Verification items for this drawing (mm, ordinates from the low corner). A direction names the side the tool comes from. Give positions to 0.01 mm unless a question says otherwise; leave off trailing zeros. Loops run counter-clockwise (first coordinate to the right, second up) from the corner with the lowest first, then second, coordinate; pieces in that order, holes last. Notation, with made-up numbers: (-10, 20.5) - (18, 20.5) arc R19 ccw to (18, 41.5) - close; hole circle Ø5 at (52, 78.25). An arc over 180 degrees is marked (long way). Write item = value, one per line. Start each with the question number.
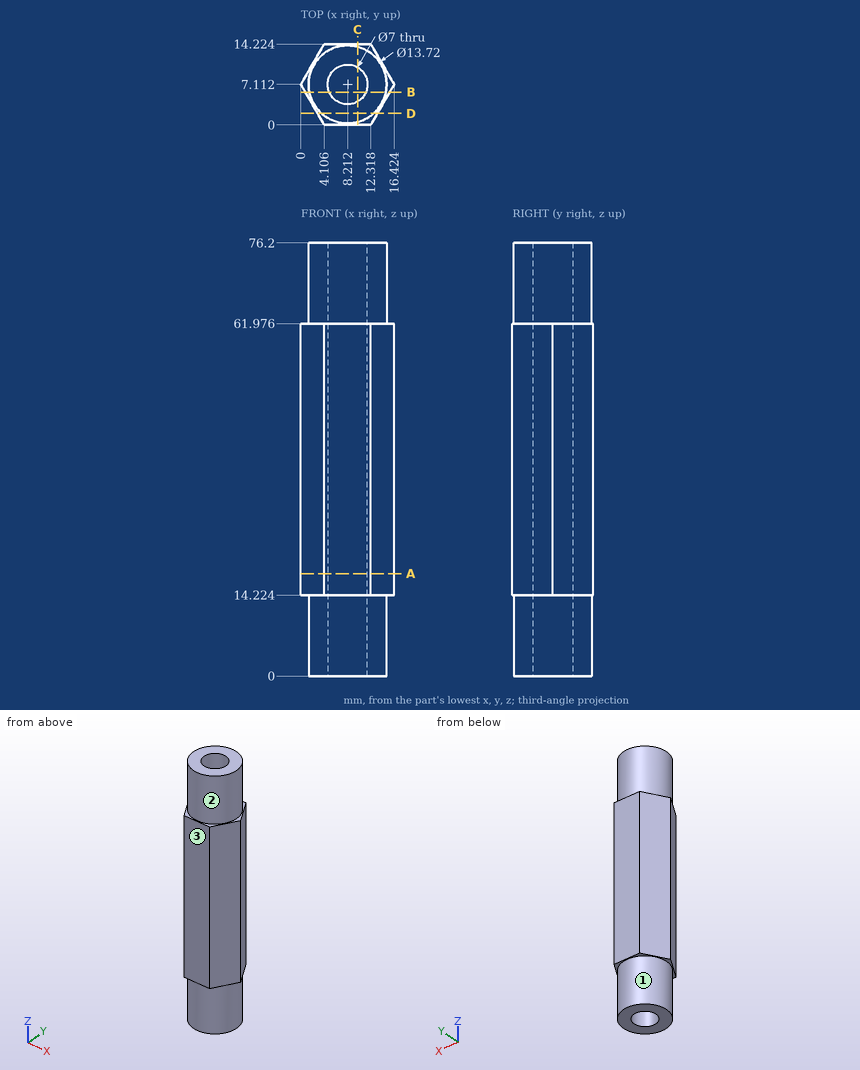
1) Cross-section at A-A on z = 18. Enter the section's corners in (x, y) (1 decimal).
2) Cross-section at B-B on y = 5.75. Enter the section's corners in (x, z) (1 decimal).
3) Gauge pin test, flat ends, axial feed: P1, Ø7, axis at x = 12, y = 8.5, coming from the -Z side; P2, Ø4, axis at y = 3, z = 42, coming from the +X side (1 decimal); P3, Ø1, axis at y = 4.5, z = 52, coming from the -X side; P4, Ø1.5, axis at y = 12, z = 25, coming from the -X side. Record the tip position at first contact, or that the pin passes through.
4) Cross-section at C-C on x = 10. Enter the section's corners in (y, z) (1 decimal).
5) Cross-section at D-D on y = 2. Enter the section's corners in (x, z).
6) Material ranges on line 1 along Y through (x, z) = (8.5, 70) (1 decimal); line 2 along Y through (x, z) = (9, 70.5); line 3 along Z through (x, y) = (15, 4.75), recorded low to high.
7) Tool access check on the marked faces 1, 2 and 3. Record the directions out of +Z, -Z, +X, -X, +Y, -Y that give a thin tool (end or side, any length) a straight path to the whole face; none if there is none.
Checked values:
q1.outline = (0, 7.1) - (4.1, 0) - (12.3, 0) - (16.4, 7.1) - (12.3, 14.2) - (4.1, 14.2) - close; hole circle Ø7 at (8.2, 7.1)
q2.outline = (0.8, 14.2) - (1.5, 14.2) - (1.5, 0) - (5, 0) - (5, 76.2) - (1.5, 76.2) - (1.5, 62) - (0.8, 62) - close; (11.4, 0) - (14.9, 0) - (14.9, 14.2) - (15.6, 14.2) - (15.6, 62) - (14.9, 62) - (14.9, 76.2) - (11.4, 76.2) - close
q3.P1 = 0
q3.P2 = 15.2
q3.P3 = 1.22
q3.P4 = 2.39
q4.outline = (0, 14.2) - (0.5, 14.2) - (0.5, 0) - (4.1, 0) - (4.1, 76.2) - (0.5, 76.2) - (0.5, 62) - (0, 62) - close; (10.1, 0) - (13.7, 0) - (13.7, 14.2) - (14.2, 14.2) - (14.2, 62) - (13.7, 62) - (13.7, 76.2) - (10.1, 76.2) - close
q5.outline = (2.95, 14.22) - (3.64, 14.22) - (3.64, 0) - (12.79, 0) - (12.79, 14.22) - (13.47, 14.22) - (13.47, 61.98) - (12.79, 61.98) - (12.79, 76.2) - (3.64, 76.2) - (3.64, 61.98) - (2.95, 61.98) - close
q6.line_1 = 0.3 to 3.6, 10.6 to 14
q6.line_2 = 0.3 to 3.7, 10.52 to 13.93
q6.line_3 = 14.22 to 61.98
q7.face_1 = -Z
q7.face_2 = +Z
q7.face_3 = +Z, -Z, +X, -X, -Y
